Autodesk Inventor part; units mm, degrees
ref_plane "YZ Plane" through (0, 0, 0) normal (1, 0, 0) x (0, 1, 0)
ref_plane "XZ Plane" through (0, 0, 0) normal (0, 1, 0) x (-1, 0, 0)
ref_plane "XY Plane" through (0, 0, 0) normal (0, 0, 1) x (1, 0, 0)
sketch "Sketch1" plane through (0, 0, 0) normal (0, 0, 1) x (1, 0, 0)
  line L0 (-490, 50) -> (490, 50)
  line L1 (490, 50) -> (490, 0)
  line L2 (490, 0) -> (-490, 0)
  line L3 (-490, 0) -> (-490, 50)
  point P0 (0, 0)
  point P1 (0, 0)
  dimension "d0" = 980
  dimension "d1" = 50
extrude "Plate1" add sketch "Sketch1" along normal blind 2
sketch "Sketch2" plane through (490, 2, 0) normal (0, -1, 0) x (1, 0, 0)
  line L0 (-980, 0) -> (0, 0)
  line L1 (0, 0) -> (0, 20)
  line L2 (0, 20) -> (-980, 20)
  line L3 (-980, 20) -> (-980, 0)
edge flange "Flange1" height 20 angle 90 thickness 2 bend radius 2.75 thickness toward (0, -1, 0) relief tear relief width 2 relief depth 1 edges at (0, 0, 2) wall of the first edge with corners at (-490, 2, 0) (490, 2, 0) (490, 2, 20) (-490, 2, 20)
bend "Bend1"
corner "Corner1"
sketch "Sketch5" plane through (0, 0, 0) normal (0, 0, -1) x (-1, 0, 0)
  line L0 (490, 50) -> (-490, 50)
  line L1 (490, 0) -> (-490, 0)
  circle A0 centre (0, 50) radius 30
  line L2 (-490, 0) -> (-490, 50)
  line L3 (490, 0) -> (490, 50)
  circle A1 centre (-490, 50) radius 30
  circle A2 centre (490, 50) radius 30
  line L4 (-246, 50) -> (-244, 50)
  line L5 (-244, 50) -> (-244, 21)
  line L6 (-244, 21) -> (-246, 21)
  line L7 (-246, 21) -> (-246, 50)
  line L8 (244, 50) -> (246, 50)
  line L9 (246, 50) -> (246, 21)
  line L10 (246, 21) -> (244, 21)
  line L11 (244, 21) -> (244, 50)
  line L12 (0, 50) -> (0, 0) construction
  point P0 (245, 21)
  point P1 (-245, 21)
  point P2 (-490, 20)
  point P3 (-460, 50)
  point P4 (-30, 50)
  point P5 (30, 50)
  point P6 (460, 50)
  point P7 (490, 20)
  point P8 (-244, 50)
  point P9 (246, 50)
  dimension "d33" = 60
  dimension "d34" = 2
  dimension "d35" = 29
  dimension "d36" = 490
extrude "Extrusion1" cut sketch "Sketch5" against normal through all contours L9 L10 L11 L0 | L0 L3 A2 | A0 L0 | L5 L6 L7 L0 | L2 L0 A1 picked at (470.2507, 47.7748) picked at (6.5355, 34.7298) picked at (-470.2507, 47.7748)
sketch "Sketch7" plane through (0, 0, 2) normal (0, 0, 1) x (1, 0, 0)
  line L0 (468.7934, 20.88) -> (468.7934, 8.88) construction
  line L1 (468.7934, 8.88) -> (280.354, 8.88) construction
  line L2 (280.354, 8.88) -> (280.354, 20.88) construction
  line L3 (280.354, 20.88) -> (468.7934, 20.88) construction
  line L4 (-244, 50) -> (-30, 50)
  point P0 (0, 0)
  point P1 (-1, 50)
  point P2 (1, 50)
  dimension "d30" = 12
mark "Mark1"
sketch "Sketch8" plane through (0, 0, 0) normal (0, 0, -1) x (-1, 0, 0)
  line L0 (-244, 50) -> (-51.6572, 50)
  line L1 (-51.6572, 50) -> (502.6857, 50)
  line L2 (502.6857, 50) -> (502.6857, -31.7842)
  line L3 (502.6857, -31.7842) -> (-51.6572, -31.7842)
  line L4 (-51.6572, -31.7842) -> (-51.6572, 50)
  point P0 (0, 0)
extrude "Extrusion3" cut sketch "Sketch8" along normal through all both and the other way through all
equation "\"d1\" = Стрингер_7"
equation "\"d2\" = Thickness"
equation "\"d3\" = BendReliefWidth"
equation "\"d4\" = BendReliefDepth"
equation "\"d5\" = MinimumRemnant"
equation "\"d6\" = TransitionRadius"
equation "\"d9\" = BendRadius"
equation "\"d10\" = CornerReliefSize"
equation "\"d11\" = GapSize"
equation "\"d12\" = JacobiRadiusSize"
equation "\"BendReliefWidth\" = Thickness"
equation "\"BendReliefDepth\" = 0.5 * Thickness"
equation "\"CornerReliefSize\" = 4 * Thickness"
equation "\"MinimumRemnant\" = 2 * Thickness"
equation "\"TransitionRadius\" = BendRadius"
equation "\"JacobiRadiusSize\" = BendRadius"
equation "\"GapSize\" = Thickness"
equation "\"Стрингер_7\" = 50"
properties part number "MSC 505 STRINGER BOARD BELLY FACE" material "Stainless Steel"
CAD build for the part. Positions are in the model's coordinates, mm. A direction names the side the tool comes from. Give positions to 0.01 mm unless a question says otherwise; leave off trailing zeros. Order: outer loops, then holes, each group sorted by start corner. A loop starts at its lowest first (then second) coordinate and runs counter-clockwise, first axis right, second up.
(1) Saw through at B-B, the plane x = 437. Give the cut face in (y, z).
(2) Saw through at C-C, the plane z = 15.5. Give the cut face in (x, y).
(3) Tool access for faces 1 (the flat face through (268, 28, 2)), 2 (the flat face through (274, 0, 12)): list every direction of +Z, -Z, +X, -X, +Y, -Y with a clear straight run to the whole face (end or side of a thin tool).
(4) Flat gauge pins, fed straight in: pin 1 (1.5 mm diameter, centred on x = 423, y = 21.5, fed in from +Z); pin 2 (10 mm diameter, centred on x = 309.5, z = 13.5, fed in from -Y); pin 3 (0.6 mm diameter, centred on x = 244.5, z = 1, fed in from +Y); pin 4 (12 mm diameter, centred on x = 254, z = 11, fed in from +Y). Where does each tip first touch, or does it go through?
(5) Drill centre lines: L1, parallel to Y at x = 380, z = 4.25; L2, parallel to Z at x = 190.5, y = 30; L3, parallel to Y at x = 146.5, z = 3.25. Where is each one in solid material? Low to high.
(6) Saw through at A-A, the plane y = 32. Give the cut face in (x, z).
Results found:
1. outline: (0, 4.75) arc R4.75 ccw to (4.75, 0) - (50, 0) - (50, 2) - (4.75, 2) arc R2.75 cw to (2, 4.75) - (2, 20) - (0, 20) - close
2. outline: (51.66, 0) - (490, 0) - (490, 2) - (51.66, 2) - close
3. face 1: +Z, +X, -X, +Y
3. face 2: +Z, -Z, +X, -X, -Y
4. pin 1: stops at z = 2
4. pin 2: stops at y = 0
4. pin 3: stops at y = 21
4. pin 4: stops at y = 2
5. L1: y = 0.03 to 2.05
5. L2: z = 0 to 2
5. L3: y = 0.24 to 2.45
6. outline: (51.66, 0) - (244, 0) - (244, 2) - (51.66, 2) - close; (246, 0) - (466, 0) - (466, 2) - (246, 2) - close
